Here's how the part is built. I have some questions about the finished solid (model axes, mm). Face numbers are marked on the shaded views. Give positions to 0.01 mm unless a question says otherwise; leave off trailing zeros. Order: outer loops, then holes, each group sorted by start corner. A loop starts at its lowest first (then second) coordinate and runs counter-clockwise, first axis right, second up. Notation, with made-up numbers: M 6,78 L 63,78 A11 cw 63,99 Z; hole C 30,70 d9. An arc over 180 degrees is marked long. Use CSV: the item, a comma, the result in double quotes. Start each with the question number.
Autodesk Inventor part; units mm, degrees
ref_plane "YZ Plane" through (0, 0, 0) normal (1, 0, 0) x (0, 1, 0)
ref_plane "XZ Plane" through (0, 0, 0) normal (0, 1, 0) x (-1, 0, 0)
ref_plane "XY Plane" through (0, 0, 0) normal (0, 0, 1) x (1, 0, 0)
sketch "main" plane through (0, 0, 0) normal (0, 0, 1) x (1, 0, 0)
  circle A0 centre (37.6731, -16.4179) radius 2.0955
  circle A1 centre (37.6731, 21.6821) radius 2.0955
  circle A2 centre (24.9731, 28.0321) radius 2.1844
  circle A3 centre (24.9731, -22.7679) radius 2.1844
  circle A4 centre (-38.5364, -16.421) radius 2.0955
  circle A5 centre (-38.5364, 21.679) radius 2.0955
  circle A6 centre (-25.8269, -10.0679) radius 2.1844
  circle A7 centre (-25.8269, 15.3321) radius 2.1844
  arc A8 (-27.9546, 11.0714) -> (-24.6718, 10.7118) centre (-25.8269, 15.3321) ccw
  arc A9 (27.103, 32.2919) -> (23.818, 32.6525) centre (24.9731, 28.0321) ccw
  arc A10 (42.4356, 21.6821) -> (39.803, 25.9419) centre (37.6731, 21.6821) ccw
  arc A11 (39.803, -20.6776) -> (42.4356, -16.4179) centre (37.6731, -16.4179) ccw
  arc A12 (23.818, -27.3882) -> (27.103, -27.0276) centre (24.9731, -22.7679) ccw
  arc A13 (-24.6718, -5.4475) -> (-27.9563, -5.8079) centre (-25.8269, -10.0679) ccw
  arc A14 (-43.2989, -16.421) -> (-36.4069, -20.6809) centre (-38.5364, -16.421) ccw
  arc A15 (-36.4086, 25.9397) -> (-43.2989, 21.679) centre (-38.5364, 21.679) ccw
  line L0 (-43.2989, 21.679) -> (-43.2989, -16.421)
  line L1 (-36.4069, -20.6809) -> (-25.273, -15.1154)
  line L2 (-36.4086, 25.9397) -> (-25.2741, 20.3794)
  line L3 (-25.2741, 20.3794) -> (23.818, 32.6525)
  line L4 (27.103, 32.2919) -> (39.803, 25.9419)
  line L5 (39.803, -20.6776) -> (27.103, -27.0276)
  line L6 (-25.273, -15.1154) -> (23.818, -27.3882)
  line L7 (-27.9546, 11.0714) -> (-29.1804, 11.6835)
  line L8 (-33.7739, 8.843) -> (-33.7739, -3.5793)
  line L9 (-29.1792, -6.4192) -> (-27.9563, -5.8079)
  line L10 (-24.6718, -5.4475) -> (24.419, -17.7203)
  line L11 (24.419, -17.7203) -> (35.5433, -12.1581)
  line L12 (35.5433, 17.4224) -> (24.419, 22.9846)
  line L13 (24.419, 22.9846) -> (-24.6718, 10.7118)
  arc A16 (-33.7739, -3.5793) -> (-29.1792, -6.4192) centre (-30.5989, -3.5793) ccw
  arc A17 (-29.1804, 11.6835) -> (-33.7739, 8.843) centre (-30.5989, 8.843) ccw
  arc A18 (35.5433, 17.4224) -> (39.803, 25.9419) centre (37.6731, 21.6821) ccw
  arc A19 (39.803, -20.6776) -> (35.5433, -12.1581) centre (37.6731, -16.4179) ccw
  point P0 (-0.4291, 2.6313)
  point P1 (-25.8269, -22.7679)
  dimension "d9" = 9.525
  dimension "d10" = 9.525
  dimension "d11" = 9.525
  dimension "d12" = 9.525
  dimension "d13" = 9.525
  dimension "d14" = 9.525
  dimension "d15" = 9.525
  dimension "d16" = 9.525
  dimension "d17" = 9.525
  dimension "d20" = 12.7
  dimension "d21" = 25.4
  dimension "d22" = 3.175
sketch "Sketch1" plane through (0, 0, 0) normal (0, 0, 1) x (1, 0, 0)
  circle A0 centre (63.5, -6.35) radius 2.0955
  circle A1 centre (63.5, 31.75) radius 2.0955
  circle A2 centre (50.8, 38.1) radius 2.1844
  circle A3 centre (50.8, -12.7) radius 2.1844
  circle A4 centre (-12.7095, -6.3532) radius 2.0955
  circle A5 centre (-12.7095, 31.7468) radius 2.0955
  circle A6 centre (0, 0) radius 2.1844
  circle A7 centre (0, 25.4) radius 2.1844
  arc A8 (-2.1277, 21.1392) -> (1.1551, 20.7797) centre (0, 25.4) ccw
  arc A9 (52.9299, 42.3597) -> (49.6449, 42.7203) centre (50.8, 38.1) ccw
  arc A10 (68.2625, 31.75) -> (65.6299, 36.0097) centre (63.5, 31.75) ccw
  arc A11 (65.6299, -10.6097) -> (68.2625, -6.35) centre (63.5, -6.35) ccw
  arc A12 (49.6449, -17.3203) -> (52.9299, -16.9597) centre (50.8, -12.7) ccw
  arc A13 (1.1551, 4.6203) -> (-2.1294, 4.2599) centre (0, 0) ccw
  arc A14 (-17.472, -6.3532) -> (-10.58, -10.6131) centre (-12.7095, -6.3532) ccw
  arc A15 (-10.5818, 36.0076) -> (-17.472, 31.7468) centre (-12.7095, 31.7468) ccw
  line L0 (-17.472, 31.7468) -> (-17.472, -6.3532)
  line L1 (-10.58, -10.6131) -> (0.5538, -5.0475)
  line L2 (-10.5818, 36.0076) -> (0.5528, 30.4473)
  line L3 (0.5528, 30.4473) -> (49.6449, 42.7203)
  line L4 (52.9299, 42.3597) -> (65.6299, 36.0097)
  line L5 (65.6299, -10.6097) -> (52.9299, -16.9597)
  line L6 (0.5538, -5.0475) -> (49.6449, -17.3203)
  line L7 (-2.1277, 21.1392) -> (-3.3535, 21.7513)
  line L8 (-7.947, 18.9108) -> (-7.947, 6.4886)
  line L9 (-3.3524, 3.6486) -> (-2.1294, 4.2599)
  line L10 (1.1551, 4.6203) -> (50.2459, -7.6524)
  line L11 (50.2459, -7.6524) -> (61.3701, -2.0903)
  line L12 (61.3701, 27.4903) -> (50.2459, 33.0524)
  line L13 (50.2459, 33.0524) -> (1.1551, 20.7797)
  arc A16 (-7.947, 6.4886) -> (-3.3524, 3.6486) centre (-4.772, 6.4886) ccw
  arc A17 (-3.3535, 21.7513) -> (-7.947, 18.9108) centre (-4.772, 18.9108) ccw
  arc A18 (61.3701, 27.4903) -> (65.6299, 36.0097) centre (63.5, 31.75) ccw
  arc A19 (65.6299, -10.6097) -> (61.3701, -2.0903) centre (63.5, -6.35) ccw
  point P0 (68.2625, -6.35)
  point P1 (68.2625, 31.75)
extrude "Extrusion1" add sketch "Sketch1" along normal blind 1.5875
properties part number "Brain Mount" material "Acetal Resin, White"
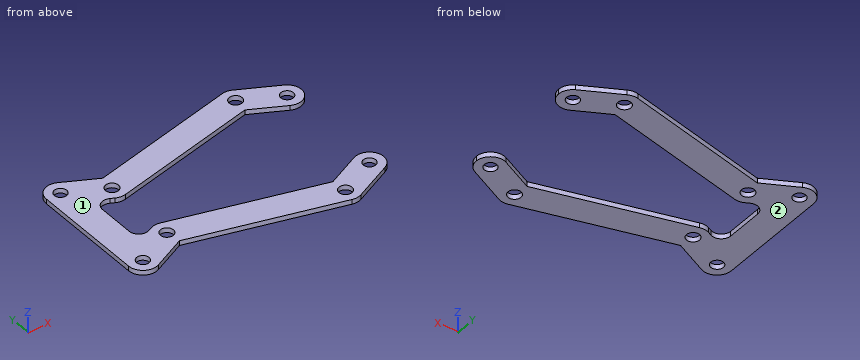
Q1. For P1, Ø2.5, axis at x = 50.8, y = -12.7, coming from the +Z side, with a flat end and sliding along its axis, tell me the tip position at first contact or that it passes through.
Q2. I need wall thicknesses on line 1 (Y direction, x = 0, z = 0.9); line 2 (Y direction, x = 50.8, z = 0.65); line 3 (Y direction, x = 38, z = 1.3). Which ranges of each line are inside material? Lowest first, please. Write a range as [from, to].
Q3. Imagine slicing it at D-D, the plane x = 39.5. Please give me the cut outline in (y, z), then the cut area to 3 significant figures.
Q4. We'd pull the mould along Z, two halves only. Please class the marked faces 1 and 2: pulls with the +Z half, pulls with the -Z half, needs draft (parallel to the pull), parting line crosses it, or undercut.
Q5. Imagine slicing it at C-C, the plane x = 63.5. Please give me the cut outline in (y, z).
Q6. Imagine slicing it at A-A, the plane z = 1.3. Count the separate pieces of the cut face and the enclosed holes in it, then the cut area to 3 significant figures.
Q7. Imagine slicing it at B-B, the plane y = 25.4. Please give me the cut outline in (x, z).
Reply:
1,P1,"passes through"
2,line 1,"y = [-5.32, -2.18], [2.18, 4.76], [20.64, 23.22], [27.58, 30.72]"
2,line 2,"y = [-17.46, -14.88], [-10.52, -7.38], [32.78, 35.92], [40.28, 42.86]"
2,line 3,"y = [-14.41, -4.59], [29.99, 39.81]"
3,outline,"M -14.78,0 L -4.97,0 L -4.97,1.59 L -14.78,1.59 Z; M 30.37,0 L 40.18,0 L 40.18,1.59 L 30.37,1.59 Z"
3,area,"31.2 mm^2"
4,face 1,"pulls with the +Z half"
4,face 2,"pulls with the -Z half"
5,outline,"M -11.67,0 L -8.45,0 L -8.45,1.59 L -11.67,1.59 Z; M -4.25,0 L -1.59,0 L -1.59,1.59 L -4.25,1.59 Z; M 26.99,0 L 29.65,0 L 29.65,1.59 L 26.99,1.59 Z; M 33.85,0 L 37.07,0 L 37.07,1.59 L 33.85,1.59 Z"
6,separate pieces,"1"
6,enclosed holes,"8"
6,area,"1,840 mm^2"
7,outline,"M -17.47,0 L -2.18,0 L -2.18,1.59 L -17.47,1.59 Z; M 2.18,0 L 19.64,0 L 19.64,1.59 L 2.18,1.59 Z"
